Build history of the part. All positions in model axes, mm. Coordinates: 2 decimals unless noted, no trailing zeros. Write each loop counter-clockwise with the first axis right and the second up, starting at its lowest first coordinate (ties: lowest second). Pieces come first, ordered by that corner, then holes.
from build123d import *

# Parameters (mm, degrees)
F1_DEPTH = 3
F4_W     = 60
F4_H     = 120
F5_DEPTH = 3


with BuildPart() as f1:
    # F0 (on Top) → F1 (new body)
    with BuildSketch(Plane.XY):
        with BuildLine():
            Line((64, 0), (64, 57.4883735822))
            Line((64, 57.4883735822), (62.8046343071, 58.8159616805))
            Line((62.8046343071, 58.8159616805), (58.717337767, 55.1357433455))
            Line((58.717337767, 55.1357433455), (57.7064563618, 56.2584408851))
            Line((57.7064563618, 56.2584408851), (64.0975018609, 62.0129640998))
            add(Edge.make_bspline(
                [(64.0975018609, 62.0129640998), (64.2947499686, 61.8134944285), (64.7475356166, 61.0205339905), (65.2331012875, 62.6495131608), (65.0931958217, 63.4477440608)],
                knots=[0, 0, 0, 0, 0.3763533344, 1, 1, 1, 1], degree=3))
            Line((65.0931958217, 63.4477440608), (63.3534562452, 65.379920607))
            Line((63.3534562452, 65.379920607), (55.6990645427, 58.4878753615))
            Line((55.6990645427, 58.4878753615), (55.3495648702, 59.0087018934))
            Line((55.3495648702, 59.0087018934), (58.971833562, 63.1474419824))
            Line((58.971833562, 63.1474419824), (58.1506918082, 64.0594122905))
            Line((58.1506918082, 64.0594122905), (60.7529463893, 66.4024928396))
            ThreePointArc((60.7529463893, 66.4024928396), (60.8269606084, 67.8147682715), (59.4146851766, 67.8887824906))
            Line((59.4146851766, 67.8887824906), (56.8124305955, 65.5457019415))
            Line((56.8124305955, 65.5457019415), (55.9912888418, 66.4576722496))
            Line((55.9912888418, 66.4576722496), (51.4965910242, 63.2878628661))
            Line((51.4965910242, 63.2878628661), (51.0151502982, 63.6898891399))
            Line((51.0151502982, 63.6898891399), (58.6695420007, 70.5819343854))
            Line((58.6695420007, 70.5819343854), (56.9298024241, 72.5141109316))
            add(Edge.make_bspline(
                [(55.3988039783, 71.673846831), (55.2210450643, 71.8908646511), (54.4797575345, 72.424056828), (56.1505684198, 72.7366878299), (56.9298024241, 72.5141109316)],
                knots=[0, 0, 0, 0, 0.3763533344, 1, 1, 1, 1], degree=3))
            Line((55.3988039783, 71.673846831), (49.0077584792, 65.9193236163))
            Line((49.0077584792, 65.9193236163), (47.996877074, 67.0420211559))
            Line((47.996877074, 67.0420211559), (52.0841736141, 70.7222394909))
            Line((52.0841736141, 70.7222394909), (50.9930178895, 71.9340906943))
            Line((50.9930178895, 71.9340906943), (0, 72))
            Line((0, 72), (0, 0))
            Line((0, 0), (64, 0))
        make_face()
        Polygon((61.6300208296, 60.8677403836), (57.1711518767, 56.8529567455), (56.2343690278, 57.8933595012), (60.6932379807, 61.9081431393), align=None, mode=Mode.SUBTRACT)
        Polygon((50.4798458131, 64.2844050003), (49.5430629642, 65.3248077559), (54.0019319171, 69.3395913941), (54.938714766, 68.2991886384), align=None, mode=Mode.SUBTRACT)
    extrude(amount=F1_DEPTH)

    # F2: F1 across face


with BuildPart() as f1_1:
    add(f1.part)
    add(f1.part.mirror(Plane(origin=(0, 36, 1.5), x_dir=(0, -1, 0), z_dir=(-1, 0, 0))))

    # F3: F1 across face


with BuildPart() as f1_2:
    add(f1_1.part)
    add(f1_1.part.mirror(Plane(origin=(0, 0, 1.5), x_dir=(1, 0, 0), z_dir=(0, -1, 0))))

    # F4 (on face) → F5 (cut)
    with BuildSketch(Plane.XY.offset(3)):
        Rectangle(F4_W, F4_H)
    extrude(amount=-F5_DEPTH, mode=Mode.SUBTRACT)


solid = f1_2.part
(1) Slice it at C-C, the plane z = 2.2. Give the number of separate pieces and of enclosed holes in the cut face, and give its area (3 significant figures).
(2) Two-plate mould, pull along Y, no slides. Class faces 1 (the flat face through (-59.432, -58.888, 1.479)), 2 (the flat face through (-43, -1, 0)): pulls with the +Y half, pulls with the -Y half, needs draft (parallel to the pull), parting line crosses it, or undercut.
(3) Slice it at A-A, the plane x = -3.5. List the corners of the cut face in (y, z).
(4) Flat gauge pins, fed straight in: P1, Ø0.9, axis at x = 4.5, z = 2, coming from the -Y side; P2, Ø1.5, axis at y = 4, z = 1, coming from the -X side; P3, Ø10, axis at x = -50, y = -14, coming from the -Z side; P4, Ø0.9, axis at y = 21.5, z = 2, coming from the +X side. Where does each tip first touch, or does it go through?
(5) Probe L1, parallel to Y at x = 7, z = 1.8; L2, parallel to X at y = 53, z = 0.45; L3, parallel to X at y = 57.5, z = 1.75. List the from-to ranges inside material, lowest first.
(6) Slice it at B-B, the plane y = -7.5. List the corners of the cut face in (x, z).
Results:
1. separate pieces: 1
1. enclosed holes: 9
1. area: 10,800 mm2
2. face 1: undercut
2. face 2: needs draft
3. outline: (-72, 0) - (-60, 0) - (-60, 3) - (-72, 3) - close; (60, 0) - (72, 0) - (72, 3) - (60, 3) - close
4. P1: stops at y = -71.99
4. P2: stops at x = -64
4. P3: stops at z = 0
4. P4: stops at x = 64
5. L1: y = -71.99 to -60, 60 to 71.99
5. L2: x = -64 to -30, 30 to 64
5. L3: x = -63.99 to -61.34, -59.09 to -57.89, -56.59 to -30, 30 to 56.59, 57.89 to 59.09, 61.34 to 63.99
6. outline: (-64, 0) - (-30, 0) - (-30, 3) - (-64, 3) - close; (30, 0) - (64, 0) - (64, 3) - (30, 3) - close
